Design review of the part built by this model. Coordinates are the model's own, in mm. A direction names the side the tool comes from. Give positions to 0.01 mm unless a question says otherwise; leave off trailing zeros. Write each loop counter-clockwise with the first axis right and the second up, starting at its lowest first coordinate (ties: lowest second). Pieces come first, ordered by that corner, then holes. Notation, with made-up numbers: (-13, 34.5) -> (13, 34.5) arc R11 cw to (13, 45.5) -> close; hole circle Ø4 at (28, -27). An arc over 180 degrees is marked (long way). Write each question's results on one line, items separated by ' | '. Start each with the question number.
(1) Clearance check with flat-ended pins moving along their axes: pin 1 (4 mm diameter, centred on x = -11, y = 11, fed in from +Z) (3 decimals); pin 2 (2.5 mm diameter, centred on x = 1.5, z = 3.5, fed in from +Y); pin 3 (1 mm diameter, centred on y = -12, z = 5.5, fed in from -X). State where each tip first meets the part, or that it passes through.
(2) For faces 1 (the face through (-3.969, 18, 5)), 2 (the face through (-10, 10, 3.175)), 3 (the face through (-10, -10, 6.35)), list the 3-axis set-ups (+Z, -Z, +X, -X, +Y, -Y) from which the entire face can be reached by the end or side of a thin tool; tool diameter is ignored.
(3) To check wall thickness, follow probe 1 along X at (y, z) = (-3, 2.5); probe 2 along X at (y, z) = (7, 3.25); probe 3 along Y at (x, z) = (4, 6.25). State the ranges of each line that lie inside material, in increasing order.
(4) Take a section at C-C (x = 12). State the section outline as (y, z) points (3 decimals).
(5) Take a section at B-B (z = 9). Count the separate pieces of the cut face and the enclosed holes in it, plus the area to 3 significant figures.
(6) Take a section at A-A (y = 4.5). State the section outline as (x, z) points (3 decimals).
(7) Take a section at D-D (x = 1). State the section outline as (y, z) points (1 decimal).
from build123d import *

# Parameters (mm, degrees)
F0_R             = 2.15265
F1_DEPTH         = 9.525
F2_R             = 2.15265
F3_REACH         = 42.6021136501
F6_R             = 3.96875
F7_DEPTH         = 6.35
F8_R             = 3.96875
F9_DEPTH         = 6.35
F11_DEPTH        = 9.525
F11_COPIES_COUNT = 3
F11_COPIES_ANGLE = 180


# Not quite as in the source:
# - a pattern or mirror of a feature is missing from the dataset's text; its kind, count and spacing are read off the source's solid


with BuildPart() as f1:
    # F0 (on Top) → F1 (new body)
    with BuildSketch(Plane.XY):
        with BuildLine():
            Line((3.96875, 14.2875), (0, 14.2875))
            Line((0, 14.2875), (-3.96875, 14.2875))
            Line((-3.96875, 14.2875), (-3.96875, 21.8677764859))
            ThreePointArc((-3.96875, 21.8677764859), (0, -22.225), (3.96875, 21.8677764859))
            Line((3.96875, 21.8677764859), (3.96875, 14.2875))
        make_face()
        with Locations((-11.7865861589, -11.7865861589)):
            Circle(F0_R, mode=Mode.SUBTRACT)
        with Locations((11.7865861589, -11.7865861589)):
            Circle(F0_R, mode=Mode.SUBTRACT)
        with Locations((-11.7865861589, 11.7865861589)):
            Circle(F0_R, mode=Mode.SUBTRACT)
        with BuildLine():
            ThreePointArc((0, 11.1125), (7.8577241059, 7.8577241059), (11.1125, 0))
            ThreePointArc((11.1125, 0), (-7.8577241059, -7.8577241059), (0, 11.1125))
        make_face(mode=Mode.SUBTRACT)
        with Locations((11.7865861589, 11.7865861589)):
            Circle(F0_R, mode=Mode.SUBTRACT)
    extrude(amount=F1_DEPTH)

    f3_end = f1.faces().sort_by_distance((0, -11.1125, 4.7625))[0]
    # F2 (on face) → F3 (cut, up to a face of the model that its end follows)
    with BuildSketch(Plane(origin=(0, 14.2875, 0), x_dir=(-1, 0, 0), z_dir=(0, 1, 0))):
        with Locations((0, 4.7625)):
            Circle(F2_R)
    f3_long = extrude(amount=-F3_REACH, mode=Mode.PRIVATE)
    add(split(f3_long, bisect_by=f3_end, keep=Keep.ALL, mode=Mode.PRIVATE).solids().sort_by_distance((0, 14.2875, 4.7625))[0], mode=Mode.SUBTRACT)

    # F6 (on face) → F7 (cut, through all)
    with BuildSketch(Plane.XY.offset(9.525)):
        with Locations((-11.7865861589, 11.7865861589)):
            Circle(F6_R)
        with Locations((11.7865861589, -11.7865861589)):
            Circle(F6_R)
    extrude(amount=-F7_DEPTH, mode=Mode.SUBTRACT)

    # F8 (on face) → F9 (cut, through all)
    with BuildSketch(Plane(origin=(0, 0, 0), x_dir=(1, 0, 0), z_dir=(0, 0, -1))):
        with Locations((11.7865861589, -11.7865861589)):
            Circle(F8_R)
        with Locations((-11.7865861589, 11.7865861589)):
            Circle(F8_R)
    extrude(amount=-F9_DEPTH, mode=Mode.SUBTRACT)

    # F10 (on face) → F11 (cut, through all)
    with BuildSketch(Plane.XY.offset(9.525)):
        with BuildLine():
            ThreePointArc((-12.8109235396, -6.3255746232), (-14.2875, 0), (-12.8109235396, 6.3255746232))
            ThreePointArc((-12.8109235396, 6.3255746232), (-15.8788163052, 8.0281867), (-17.3148424047, 11.229543123))
            ThreePointArc((-17.3148424047, 11.229543123), (-20.6375, 0), (-17.3148424047, -11.229543123))
            ThreePointArc((-17.3148424047, -11.229543123), (-15.8788163052, -8.0281867), (-12.8109235396, -6.3255746232))
        make_face()
    f11 = extrude(amount=-F11_DEPTH, mode=Mode.SUBTRACT)

    # F11_copies: F11 ×3 about axis
    f11_copies_axis = Axis((0, 0, 0), (0, 0, 1))
    for i in range(1, F11_COPIES_COUNT):
        add(f11.rotate(f11_copies_axis, i * F11_COPIES_ANGLE / (F11_COPIES_COUNT - 1)), mode=Mode.SUBTRACT)


solid = f1.part
Report:
1) pin 1: z = 3.175 | pin 2: y = 14.29 | pin 3: x = -19.02
2) face 1: +Z, -Z, +Y | face 2: +Z | face 3: -Z
3) probe 1: -22.02 to -20.42, -13.97 to -10.7, 10.7 to 13.97, 20.42 to 22.02 | probe 2: -21.09 to -19.41, -14.61 to -8.63, 8.63 to 14.61, 19.41 to 21.09 | probe 3: -21.86 to -20.25, -13.72 to -10.37, 10.37 to 21.86
4) outline: (-18.707, 0) -> (-13.929, 0) -> (-13.929, 3.175) -> (-15.75, 3.175) -> (-15.75, 9.525) -> (-18.707, 9.525) -> close; (-9.645, 0) -> (7.824, 0) -> (7.824, 6.35) -> (9.645, 6.35) -> (9.645, 9.525) -> (-7.824, 9.525) -> (-7.824, 3.175) -> (-9.645, 3.175) -> close; (13.929, 6.35) -> (15.75, 6.35) -> (15.75, 0) -> (18.707, 0) -> (18.707, 9.525) -> (13.929, 9.525) -> close
5) separate pieces: 1 | enclosed holes: 8 | area: 653 mm2
6) outline: (-21.765, 0) -> (-20.141, 0) -> (-20.141, 9.525) -> (-21.765, 9.525) -> close; (-13.56, 0) -> (-10.161, 0) -> (-10.161, 9.525) -> (-13.56, 9.525) -> close; (10.161, 0) -> (13.56, 0) -> (13.56, 9.525) -> (10.161, 9.525) -> close; (20.141, 0) -> (21.765, 0) -> (21.765, 9.525) -> (20.141, 9.525) -> close
7) outline: (-22.2, 0) -> (-20.6, 0) -> (-20.6, 9.5) -> (-22.2, 9.5) -> close; (-14.3, 0) -> (-11.1, 0) -> (-11.1, 9.5) -> (-14.3, 9.5) -> close; (11.1, 0) -> (14.3, 0) -> (14.3, 2.9) -> (11.1, 2.9) -> close; (11.1, 6.7) -> (14.3, 6.7) -> (14.3, 9.5) -> (11.1, 9.5) -> close
